Autodesk Inventor part; units mm, degrees
ref_plane "YZ Plane" through (0, 0, 0) normal (1, 0, 0) x (0, 1, 0)
ref_plane "XZ Plane" through (0, 0, 0) normal (0, 1, 0) x (-1, 0, 0)
ref_plane "XY Plane" through (0, 0, 0) normal (0, 0, 1) x (1, 0, 0)
sketch "スケッチ1" plane through (0, 0, 0) normal (0, 1, 0) x (-1, 0, 0)
  circle A0 centre (0, 0) radius 25
  dimension "d0" = 50
extrude "押し出し1" add sketch "スケッチ1" along normal blind 5
sketch "スケッチ4" plane through (0, 5, 0) normal (0, 1, 0) x (1, 0, 0)
  circle A0 centre (0, 0) radius 17.5
  dimension "d9" = 35
extrude "押し出し4" cut sketch "スケッチ4" against normal through all
chamfer "面取り2" distance 0.5 angle 45 4 edges at (25, 5, 0) (-17.5, 5, 0) (-17.5, 0, 0) (25, 0, 0)
properties part number "B_probe_bearing_clamp_without_holes" material "PAEK 樹脂"
Check sheet for the modelled part. Datum: model origin and axes. Units: mm. Give positions to 0.01 mm unless a question says otherwise; leave off trailing zeros. Order: outer loops, then holes, each group sorted by start corner. A loop starts at its lowest first (then second) coordinate and runs counter-clockwise, first axis right, second up. Notation, with made-up numbers: M 21.5,71 L 33.5,71 A29 cw 33.5,102 Z; hole C 54,72 d10. An arc over 180 degrees is marked long. Answer in a Markdown table with one row per item. Add a question column.
Q1. Sectioned sample at B-B, the plane x = 0. Record the boundary of the cut face in (y, z), and give its area (3 significant figures).
Q2. Sectioned sample at A-A, the plane z = 0. Record the boundary of the cut face in (x, y), and give its area (3 significant figures).
Q3. Sectioned sample at C-C, the plane y = 1.25. Record the boundary of the cut face in (x, z).
Q4. Release check for a two-part mould opening along X. For faces 1 (the cylindrical face through (-23.846, 2.472, -7.509)), 2 (the cylindrical face through (-13.887, 2.528, 10.648)), 3 (the flat face through (13, 5, 13)) record: released by +X, released by -X, zero draft, split by the parting line, or undercut.
Q5. Gauge pin test, flat ends, axial feed: pin 1 Ø1 at (x, y) = (9, 2) entering from -Z; pin 2 Ø10 at (x, z) = (-12.5, -2) entering from +Y; pin 3 Ø1 at (x, y) = (10.5, 4.5) entering from -Z. Record the tip position at first contact, or that the pin passes through.
Q6. Thickness scan on L1, parallel to Z at x = 0, y = 2.35; L2, parallel to Z at x = -1.5, y = 2.25; L3, parallel to X at y = 3.8, z = 11. Record the ranges inside material, lowest first.
Verdict:
| question | item | result |
|---|---|---|
| 1 | outline | M 0,-24.5 L 0.5,-25 L 4.5,-25 L 5,-24.5 L 5,-18 L 4.5,-17.5 L 0.5,-17.5 L 0,-18 Z; M 0,18 L 0.5,17.5 L 4.5,17.5 L 5,18 L 5,24.5 L 4.5,25 L 0.5,25 L 0,24.5 Z |
| 1 | area | 74.0 mm² |
| 2 | outline | M -25,0.5 L -24.5,0 L -18,0 L -17.5,0.5 L -17.5,4.5 L -18,5 L -24.5,5 L -25,4.5 Z; M 17.5,0.5 L 18,0 L 24.5,0 L 25,0.5 L 25,4.5 L 24.5,5 L 18,5 L 17.5,4.5 Z |
| 2 | area | 74.0 mm² |
| 3 | outline | C 0,0 d50; hole C 0,0 d35 |
| 4 | face 1 | split by the parting line |
| 4 | face 2 | undercut |
| 4 | face 3 | zero draft |
| 5 | pin 1 | z = -23.51 |
| 5 | pin 2 | y = 4.66 |
| 5 | pin 3 | z = -22.91 |
| 6 | L1 | -25 to -17.5, 17.5 to 25 |
| 6 | L2 | -24.95 to -17.44, 17.44 to 24.95 |
| 6 | L3 | -22.45 to -13.61, 13.61 to 22.45 |
